Part print with two shaded views. Sizes in mm from the minimum x, y, z corner. Coordinates: 2 decimals unless noted, no trailing zeros. Order: outer loops, then holes, each group sorted by start corner. A loop starts at its lowest first (then second) coordinate and runs counter-clockwise, first axis right, second up. Notation, with made-up numbers: (73, 65.5) - (112, 65.5) arc R18 ccw to (112, 95.5) - close; hole circle Ø7 at (-16, 33). An arc over 180 degrees is marked (long way). Return JSON: item names as keys, results as strings.
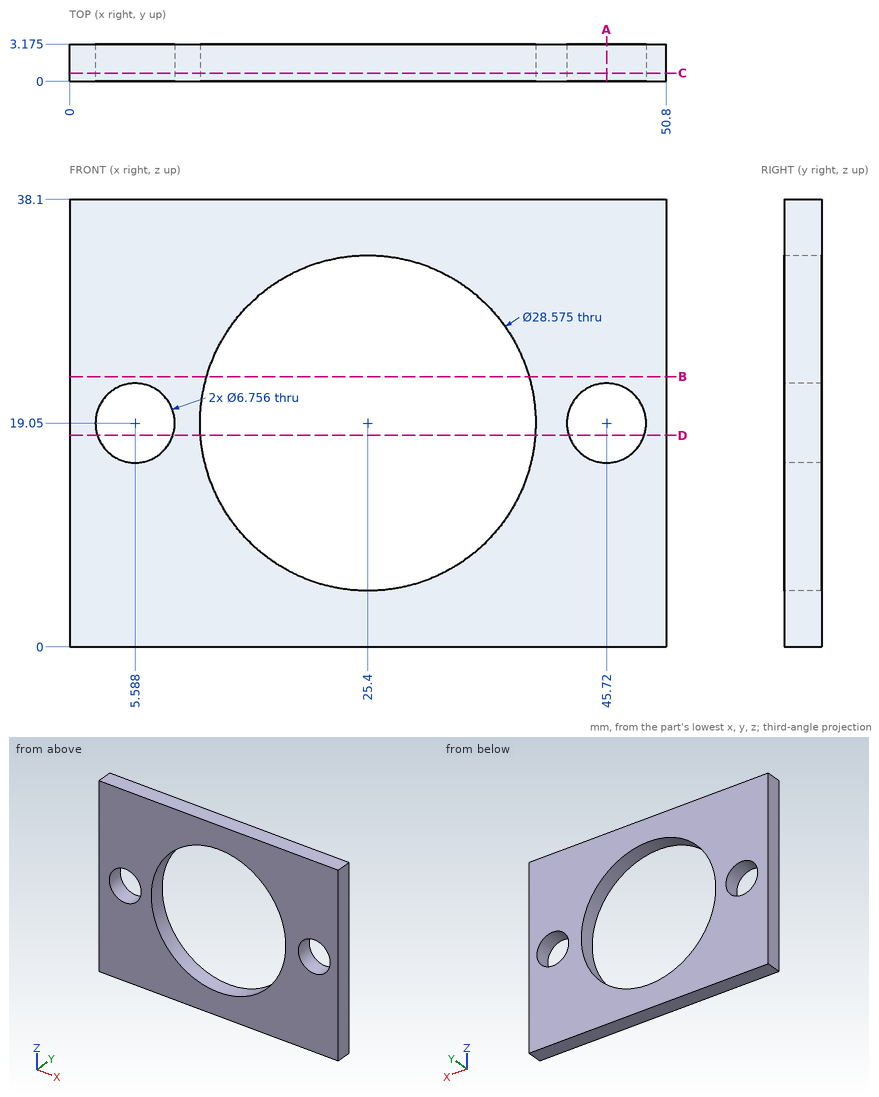
Item 1: Band-saw the part on B-B, the plane z = 23. List the corners of the cut face in (x, y) (1 decimal).
Findings below:
{"outline": "(0, 0) - (11.7, 0) - (11.7, 3.2) - (0, 3.2) - close; (39.1, 0) - (50.8, 0) - (50.8, 3.2) - (39.1, 3.2) - close"}
Item 2: Wall check: L1, parallel to X at y = 1.7, z = 19.05; L2, parallel to Z at x = 46, y = 1.85; L3, parallel to X at y = 0.95, z = 21.5 (1 decimal). Give the ranges that are in metal, low to high. Write a range as [from, to].
Findings below:
{"L1": "x = [0, 2.21], [8.97, 11.11], [39.69, 42.34], [49.1, 50.8]", "L2": "z = [0, 15.68], [22.42, 38.1]", "L3": "x = [0, 3.3], [7.9, 11.3], [39.5, 43.4], [48, 50.8]"}
Item 3: Band-saw the part on A-A, the plane x = 45.72. List the corners of the cut face in (y, z) (1 decimal).
Findings below:
{"outline": "(0, 0) - (3.2, 0) - (3.2, 15.7) - (0, 15.7) - close; (0, 22.4) - (3.2, 22.4) - (3.2, 38.1) - (0, 38.1) - close"}
Item 4: Band-saw the part on C-C, the plane y = 0.7. Count the separate pieces of the cut face and the enclosed holes in it, then the cut area to 3 significant figures.
Findings below:
{"separate pieces": "1", "enclosed holes": "3", "area": "1,220 mm²"}
Item 5: Band-saw the part on D-D, the plane z = 18. List the corners of the cut face in (x, y) (1 decimal).
Findings below:
{"outline": "(0, 0) - (2.4, 0) - (2.4, 3.2) - (0, 3.2) - close; (8.8, 0) - (11.2, 0) - (11.2, 3.2) - (8.8, 3.2) - close; (39.6, 0) - (42.5, 0) - (42.5, 3.2) - (39.6, 3.2) - close; (48.9, 0) - (50.8, 0) - (50.8, 3.2) - (48.9, 3.2) - close"}
Item 6: Drop flat-ended pins along their axis: P1, Ø1.5, axis at x = 17.5, y = 1.5, coming from the -Z side; P2, Ø4, axis at x = 45.72, z = 19.05, coming from the -Y side. Give the stop position or say it passes through.
Findings below:
{"P1": "stops at z = 0", "P2": "passes through"}
